Part print with two shaded views. Sizes in mm from the minimum x, y, z corner. Round coordinates to 2 decimals unless told otherwise and drop trailing zeros. Order: outer loops, then holes, each group sorted by start corner. A loop starts at its lowest first (then second) coordinate and runs counter-clockwise, first axis right, second up. Notation, with made-up numbers: (60.25, -25) -> (77.25, -25) arc R15 cw to (77.25, -4) -> close; hole circle Ø3 at (77.25, 67.5). An arc over 180 degrees is marked (long way). Answer as a JSON object with one key per item and string values.
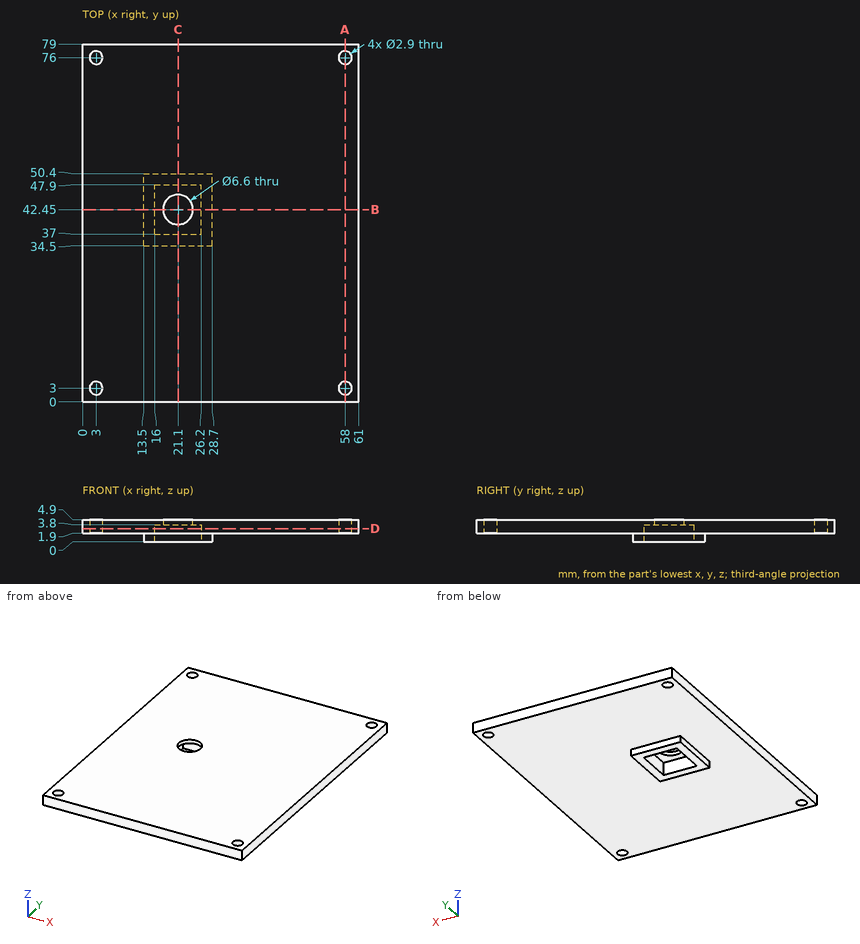
1) Cut at B-B, the plane y = 42.45. Give the cut face in (x, z), plus the area to 3 significant figures.
Checked values:
{"outline": "(0, 1.9) -> (13.5, 1.9) -> (13.5, 0) -> (16, 0) -> (16, 3.8) -> (17.8, 3.8) -> (17.8, 4.9) -> (0, 4.9) -> close; (24.4, 3.8) -> (26.2, 3.8) -> (26.2, 0) -> (28.7, 0) -> (28.7, 1.9) -> (61, 1.9) -> (61, 4.9) -> (24.4, 4.9) -> close", "area": "166 mm²"}
2) Cut at A-A, the plane x = 58. Give the cut face in (y, z), plus the area to 3 significant figures.
Checked values:
{"outline": "(0, 1.9) -> (1.55, 1.9) -> (1.55, 4.9) -> (0, 4.9) -> close; (4.45, 1.9) -> (74.55, 1.9) -> (74.55, 4.9) -> (4.45, 4.9) -> close; (77.45, 1.9) -> (79, 1.9) -> (79, 4.9) -> (77.45, 4.9) -> close", "area": "220 mm²"}
3) Probe L1, parallel to Y at x = 3, z = 3.8; L2, parallel to Y at x = 23, z = 2.95; L3, parallel to Z at x = 33, y = 53.5. List the from-to ranges inside material, lowest first. Write a range as from..to.
Checked values:
{"L1": "y = 0..1.55, 4.45..74.55, 77.45..79", "L2": "y = 0..37, 47.9..79", "L3": "z = 1.9..4.9"}
4) Cut at C-C, the plane x = 21.1. Give the cut face in (y, z), plus the area to 3 significant figures.
Checked values:
{"outline": "(0, 1.9) -> (34.5, 1.9) -> (34.5, 0) -> (37, 0) -> (37, 3.8) -> (39.15, 3.8) -> (39.15, 4.9) -> (0, 4.9) -> close; (45.75, 3.8) -> (47.9, 3.8) -> (47.9, 0) -> (50.4, 0) -> (50.4, 1.9) -> (79, 1.9) -> (79, 4.9) -> (45.75, 4.9) -> close", "area": "219 mm²"}
5) Cut at D-D, the plane z = 2.95. Give the cut face in (x, y).
Checked values:
{"outline": "(0, 0) -> (61, 0) -> (61, 79) -> (0, 79) -> close; hole circle Ø2.9 at (3, 3); hole circle Ø2.9 at (3, 76); hole (16, 37) -> (26.2, 37) -> (26.2, 47.9) -> (16, 47.9) -> close; hole circle Ø2.9 at (58, 3); hole circle Ø2.9 at (58, 76)"}
6) Flat gauge pins, fed straight in: pin 1 Ø1.1 at (x, z) = (19.5, 2) entering from -Y; pin 2 Ø6 at (x, y) = (22.5, 42) entering from -Z; pin 3 Ø0.6 at (y, z) = (44.5, 0.5) entering from -X; pin 4 Ø4 at (x, y) = (58, 76) entering from -Z. Where does each tip first touch, or does it go through?
Checked values:
{"pin 1": "stops at y = 0", "pin 2": "stops at z = 3.8", "pin 3": "stops at x = 13.5", "pin 4": "stops at z = 1.9"}
